Can you work these out from the model? Positions are in its coordinate system, mm. Give positions to 0.01 mm unless a question says otherwise; leave off trailing zeros. Loops run counter-clockwise (first coordinate to the right, second up) from the corner with the lowest first, then second, coordinate; pieces in that order, holes last. Notation, with made-up numbers: (63.25, 0.5) - (105.25, 0.5) arc R11 cw to (105.25, 8.5) - close; hole circle Ø2 at (5, 75.25). An arc over 180 degrees is marked (long way). Use a Markdown table: item, result. Add a question column.
```python
from build123d import *

# Parameters (mm, degrees)
SKETCH1_W           = 6
SKETCH1_H           = 22
SKETCH1_R           = 2
BOSS_EXTRUDE1_DEPTH = 35.7
FILLET1_R           = 3
SKETCH2_W           = 0.474893162
SKETCH2_H           = 5.291666667
CUT_EXTRUDE1_DEPTH  = 0.3


with BuildPart() as part:
    # Sketch1 → Boss-Extrude1 (new body)
    with BuildSketch(Plane(origin=(0, 0, 0), x_dir=(1, 0, 0), z_dir=(0, 1, 0))):
        with Locations((3, -11)):
            Rectangle(SKETCH1_W, SKETCH1_H)
        with Locations(Location((3, -11, 0), (0, 0, 90))):
            Circle(SKETCH1_R, mode=Mode.SUBTRACT)
        with Locations(Location((3, -19, 0), (0, 0, 90))):
            Circle(SKETCH1_R, mode=Mode.SUBTRACT)
        with Locations(Location((3, -3, 0), (0, 0, 90))):
            Circle(SKETCH1_R, mode=Mode.SUBTRACT)
    extrude(amount=BOSS_EXTRUDE1_DEPTH)

    # Fillet1
    fillet1_edges = [part.edges().sort_by_distance(p)[0] for p in [
        (0, 17.85, 0),
        (6, 17.85, 0),
        (0, 17.85, 22),
        (6, 17.85, 22),
    ]]
    fillet(fillet1_edges, radius=FILLET1_R - 0.0001)  # a hair under: the kernel refuses the full size

    # Sketch2 → Cut-Extrude1 (cut)
    # profile 1 of 2: a face of its own
    with BuildSketch(Plane(origin=(6, 0, 0), x_dir=(0, 0, -1), z_dir=(1, 0, 0))):
        with BuildLine():
            Line((-13.408386752, 21.352777778), (-12.370617989, 21.352777778))
            add(Edge.make_bspline(
                [(-12.370617989, 21.352777778), (-12.299239595, 21.352699316), (-12.162475422, 21.352548979), (-11.966358612, 21.34799097), (-11.788241518, 21.341902995), (-11.628508204, 21.333463704), (-11.486667198, 21.323490288), (-11.363360329, 21.309502086), (-11.257618381, 21.294896639), (-11.19425982, 21.280047607), (-11.165364583, 21.273275574)],
                knots=[0, 0, 0, 0, 1.415646017, 2.712440637, 3.8905458, 4.950247383, 5.884950622, 6.709939814, 7.411656543, 8, 8, 8, 8], degree=3))
            add(Edge.make_bspline(
                [(-11.165364583, 21.273275574), (-11.128786264, 21.263263817), (-11.056491549, 21.243476216), (-10.952319734, 21.203843563), (-10.853208563, 21.156850289), (-10.758817992, 21.103292666), (-10.670307938, 21.040872825), (-10.586357852, 20.972121046), (-10.507708596, 20.895449984), (-10.434802444, 20.81171958), (-10.367848048, 20.722335453), (-10.310199599, 20.625963272), (-10.261928672, 20.52422523), (-10.220527774, 20.417192092), (-10.190730468, 20.303965056), (-10.168283369, 20.18533086), (-10.154035742, 20.061302221), (-10.152671154, 19.97654504), (-10.151976496, 19.933398438)],
                knots=[0, 0, 0, 0, 0.999701418, 1.975846123, 2.934577507, 3.890451536, 4.834027766, 5.787354733, 6.749476667, 7.726910423, 8.712836071, 9.690891519, 10.682875813, 11.679750201, 12.712814741, 13.765529915, 14.8625177, 16, 16, 16, 16], degree=3))
            add(Edge.make_bspline(
                [(-10.151976496, 19.933398438), (-10.15261365, 19.88988918), (-10.153860285, 19.804760378), (-10.168822526, 19.680220568), (-10.188976506, 19.561205859), (-10.219966097, 19.447980142), (-10.260554198, 19.341215822), (-10.308167182, 19.239281341), (-10.365594663, 19.143910884), (-10.431581489, 19.054758218), (-10.504986876, 18.97173966), (-10.585500246, 18.895456816), (-10.672796558, 18.82635621), (-10.766598377, 18.764282928), (-10.867820172, 18.71067641), (-10.974926761, 18.66266239), (-11.088849112, 18.622338286), (-11.167683628, 18.601126169), (-11.207765759, 18.590341213)],
                knots=[0, 0, 0, 0, 1.121902311, 2.195077645, 3.232258892, 4.234102512, 5.217864754, 6.176164875, 7.132989551, 8.084763148, 9.034132444, 9.988522005, 10.94243251, 11.903244335, 12.886203696, 13.894208494, 14.929344452, 16, 16, 16, 16], degree=3))
            add(Edge.make_bspline(
                [(-11.207765759, 18.590341213), (-11.240917799, 18.583291229), (-11.313572424, 18.567840781), (-11.433228682, 18.550592281), (-11.57254373, 18.535869956), (-11.731327415, 18.524831331), (-11.909437212, 18.515381369), (-12.10696947, 18.507870085), (-12.324311944, 18.503742806), (-12.475912515, 18.50352994), (-12.555063101, 18.503418803)],
                knots=[0, 0, 0, 0, 0.601384939, 1.31797006, 2.144135048, 3.087295005, 4.142315834, 5.309527816, 6.595305764, 8, 8, 8, 8], degree=3))
            Line((-12.555063101, 18.503418803), (-12.93349359, 18.503418803))
            Line((-12.93349359, 18.503418803), (-12.93349359, 16.061111111))
            Line((-12.93349359, 16.061111111), (-13.408386752, 16.061111111))
            Line((-13.408386752, 16.061111111), (-13.408386752, 21.352777778))
        make_face()
        with BuildLine():
            Line((-12.93349359, 20.810042735), (-12.93349359, 19.046153846))
            Line((-12.93349359, 19.046153846), (-12.007027911, 19.034493523))
            add(Edge.make_bspline(
                [(-12.007027911, 19.034493523), (-11.961791833, 19.034470143), (-11.874464516, 19.03442501), (-11.748316893, 19.040450288), (-11.631281423, 19.047405855), (-11.523717601, 19.05758993), (-11.425576938, 19.071985165), (-11.336695793, 19.086517197), (-11.257763354, 19.107540781), (-11.165387179, 19.135848278), (-11.062451642, 19.184127352), (-10.950468563, 19.254203972), (-10.855565414, 19.343528376), (-10.773441323, 19.44396093), (-10.708269341, 19.555689376), (-10.660559686, 19.675234078), (-10.632527222, 19.801369041), (-10.628768334, 19.88768087), (-10.626869658, 19.931278379)],
                knots=[0, 0, 0, 0, 1.160613943, 2.240541288, 3.23993089, 4.169200891, 5.011653406, 5.7853311, 6.478053781, 7.106038997, 8.262395093, 9.384106736, 10.481365981, 11.59014053, 12.70357646, 13.786202915, 14.881775077, 16, 16, 16, 16], degree=3))
            add(Edge.make_bspline(
                [(-10.626869658, 19.931278379), (-10.628778659, 19.973821131), (-10.632573518, 20.058390858), (-10.660779406, 20.182334936), (-10.708176583, 20.30061987), (-10.773878815, 20.410948226), (-10.853618381, 20.511019393), (-10.946297149, 20.597949574), (-11.051696961, 20.667832386), (-11.14974131, 20.712937467), (-11.236828818, 20.740477228), (-11.312472376, 20.759746213), (-11.397880896, 20.775130761), (-11.493082182, 20.787588104), (-11.597338347, 20.798252266), (-11.711545085, 20.805488208), (-11.83526976, 20.809723743), (-11.921161933, 20.80993383), (-11.965686765, 20.810042735)],
                knots=[0, 0, 0, 0, 1.120700087, 2.227813068, 3.331159281, 4.466773991, 5.599788987, 6.693661531, 7.80175334, 8.91857717, 9.525282508, 10.207424825, 10.974604443, 11.810962634, 12.737642355, 13.736264703, 14.826523623, 16, 16, 16, 16], degree=3))
            Line((-11.965686765, 20.810042735), (-12.93349359, 20.810042735))
        make_face(mode=Mode.SUBTRACT)
    # profile 2 of 2: a face of its own
    with BuildSketch(Plane(origin=(6, 0, 0), x_dir=(0, 0, -1), z_dir=(1, 0, 0))):
        with Locations((-8.829059829, 18.706944445)):
            Rectangle(SKETCH2_W, SKETCH2_H)
    extrude(amount=-CUT_EXTRUDE1_DEPTH, mode=Mode.SUBTRACT)


solid = part.part
```
1. Suppose I cut it at A-A (y = 16.5). State how many separate pieces and enclosed holes the cut face has, and give its area (3 significant figures).
2. Suppose I cut it at C-C (x = 2.5). List the corners of the cut face in (y, z) for me, and give its area (3 significant figures).
3. Suppose I cut it at B-B (z = 2). List the corners of the cut face in (x, y) for me, and give its area (3 significant figures).
4. If we mould it in two halves opening along Z, with no side actions, what happens to faces 1 (the face through (5.1, 18.1, 21.14)), 2 (the face through (4.2, 17.6, 12.6)), 3 (the face through (0, 18, 11))? For each: released by +Z, released by -Z, zero draft, split by the parting line, or undercut.
5. Please list where these lines run through material, in increasing order: line 1 along Z through (x, y) = (1.5, 4); line 2 along Z through (x, y) = (3.75, 32.5); line 3 along X through (y, z) = (26, 19). Write a range as [from, to].
6. Will this pin go through, and if not, where does the flat tip stop? P1, Ø3, axis at x = 3, z = 11, coming from the +Y side.
Results below:
| question | item | result |
|---|---|---|
| 1 | separate pieces | 1 |
| 1 | enclosed holes | 3 |
| 1 | area | 86.3 mm² |
| 2 | outline | (0, 0.04) - (35.7, 0.04) - (35.7, 1.06) - (0, 1.06) - close; (0, 4.94) - (35.7, 4.94) - (35.7, 9.06) - (0, 9.06) - close; (0, 12.94) - (35.7, 12.94) - (35.7, 17.06) - (0, 17.06) - close; (0, 20.94) - (35.7, 20.94) - (35.7, 21.96) - (0, 21.96) - close |
| 2 | area | 368 mm² |
| 3 | outline | (0.17, 0) - (1.27, 0) - (1.27, 35.7) - (0.17, 35.7) - close; (4.73, 0) - (5.83, 0) - (5.83, 35.7) - (4.73, 35.7) - close |
| 3 | area | 78.3 mm² |
| 4 | face 1 | released by +Z |
| 4 | face 2 | undercut |
| 4 | face 3 | zero draft |
| 5 | line 1 | [0.4, 1.68], [4.32, 9.68], [12.32, 17.68], [20.32, 21.6] |
| 5 | line 2 | [0.1, 1.15], [4.85, 9.15], [12.85, 17.15], [20.85, 21.9] |
| 5 | line 3 | [0, 1], [5, 6] |
| 6 | P1 | through |
